Solid Edge part; units mm, degrees
sketch "Sketch1" plane through (0, 0, 0) normal (0, 0, 1) x (1, 0, 0)
  line L0 (-35, -27.5) -> (35, -27.5)
  line L1 (35, -27.5) -> (35, 27.5)
  line L2 (35, 27.5) -> (-35, 27.5)
  line L3 (-35, 27.5) -> (-35, -27.5)
extrude "Protrusion1" add sketch "Sketch1" along normal blind 1.6
sketch "Sketch2" plane through (0, 0, 0) normal (0, 0, 1) x (1, 0, 0)
  circle A0 centre (-31.5, -24) radius 1.5
  circle A1 centre (-31.5, 24) radius 1.5
  circle A2 centre (31.5, 24) radius 1.5
  circle A3 centre (31.5, -24) radius 1.5
extrude "Cutout1" cut sketch "Sketch2" along normal up to vertex (1.6 mm away)
sketch "Sketch3" plane through (0, 0, 1.6) normal (0, 0, 1) x (1, 0, 0)
  line L0 (-28, 17.5) -> (-46, 17.5)
  line L1 (-46, 17.5) -> (-46, 3.5)
  line L2 (-46, 3.5) -> (-28, 3.5)
  line L3 (-28, 3.5) -> (-28, 17.5)
extrude "ExtrudedProtrusion_2" add sketch "Sketch3" along normal blind 5
sketch "Sketch4" plane through (0, 0, 1.6) normal (0, 0, 1) x (1, 0, 0)
  line L0 (-35, -0.7) -> (-35, -9.7)
  line L1 (-35, -9.7) -> (-27.5, -9.7)
  line L2 (-27.5, -9.7) -> (-27.5, -0.7)
  line L3 (-27.5, -0.7) -> (-35, -0.7)
extrude "ExtrudedProtrusion_3" add sketch "Sketch4" along normal blind 3
sketch "Sketch5" plane through (0, 0, 1.6) normal (0, 0, 1) x (1, 0, 0)
  line L0 (25.5, -11.5) -> (-26.5, -11.5)
  line L1 (-26.5, -11.5) -> (-26.5, -24.5)
  line L2 (-26.5, -24.5) -> (25.5, -24.5)
  line L3 (25.5, -24.5) -> (25.5, -11.5)
extrude "ExtrudedProtrusion_4" add sketch "Sketch5" along normal blind 10
sketch "Sketch6" plane through (0, 0, 1.6) normal (0, 0, 1) x (1, 0, 0)
  line L0 (-23.5285, 7.5572) -> (-17.5285, 7.5572)
  line L1 (-17.5285, 7.5572) -> (-17.5285, 11.5572)
  line L2 (-17.5285, 11.5572) -> (-23.5285, 11.5572)
  line L3 (-23.5285, 11.5572) -> (-23.5285, 7.5572)
  line L4 (22.7373, -7.827) -> (22.7373, -3.827)
  line L5 (22.7373, -3.827) -> (16.7373, -3.827)
  line L6 (16.7373, -3.827) -> (16.7373, -7.827)
  line L7 (16.7373, -7.827) -> (22.7373, -7.827)
extrude "ExtrudedProtrusion_5" add sketch "Sketch6" along normal blind 2
sketch "Sketch7" plane through (0, 0, 1.6) normal (0, 0, 1) x (1, 0, 0)
  line L0 (13.5, 18.5) -> (-4.5, 18.5)
  line L1 (-4.5, 18.5) -> (-4.5, -7.5)
  line L2 (-4.5, -7.5) -> (13.5, -7.5)
  line L3 (13.5, -7.5) -> (13.5, 18.5)
extrude "ExtrudedProtrusion_6" add sketch "Sketch7" along normal blind 3
sketch "Sketch8" plane through (0, 0, 0) normal (0, 0, -1) x (-1, 0, 0)
  line L0 (26.5, -24.5) -> (-25.5, -24.5)
  line L1 (-25.5, -24.5) -> (-25.5, -11.5)
  line L2 (-25.5, -11.5) -> (26.5, -11.5)
  line L3 (26.5, -11.5) -> (26.5, -24.5)
extrude "ExtrudedProtrusion_7" add sketch "Sketch8" along normal blind 2
properties material "Polycarbonate"
Model file for the job. Use its own axes, mm. A direction names the side the tool comes from. Give positions to 0.01 mm unless a question says otherwise; leave off trailing zeros. Loops run counter-clockwise (first coordinate to the right, second up) from the corner with the lowest first, then second, coordinate; pieces in that order, holes last. Notation, with made-up numbers: M 49,-35 L 56,-35 A35 cw 56,3 Z; hole C 19.25,-13 d8. An arc over 180 degrees is marked long. Use one line per item in the form item = value.
Item 1: Slice it at A-A on x = 31.5. List the corners of the cut face in (y, z), and give its area (3 significant figures).
Filled in:
outline = M -27.5,0 L -25.5,0 L -25.5,1.6 L -27.5,1.6 Z; M -22.5,0 L 22.5,0 L 22.5,1.6 L -22.5,1.6 Z; M 25.5,0 L 27.5,0 L 27.5,1.6 L 25.5,1.6 Z
area = 78.4 mm^2
Item 2: Which spindle directions (+Z, -Z, +X, -X, +Y, -Y) get a long thin tool onto all of the face, cutting with end or side? Do faces 5 (the flat face through (20, -6, 3.6)), 6 (the flat face through (-28, 10, 4)), 7 (the flat face through (-31, -5, 4.6)), 8 (the flat face through (0, -11.5, -1)), 9 (the flat face through (-31, -0.7, 3)). Say none if no direction does.
Filled in:
face_5 = +Z, +X, +Y
face_6 = +Z, +Y
face_7 = +Z, +X, -X, -Y
face_8 = -Z, +X, -X, +Y
face_9 = +Z, -X
Item 3: Slice it at D-D on x = 3. List the corners of the cut face in (y, z).
Filled in:
outline = M -27.5,0 L -24.5,0 L -24.5,-2 L -11.5,-2 L -11.5,0 L 27.5,0 L 27.5,1.6 L 18.5,1.6 L 18.5,4.6 L -7.5,4.6 L -7.5,1.6 L -11.5,1.6 L -11.5,11.6 L -24.5,11.6 L -24.5,1.6 L -27.5,1.6 Z
Item 4: Slice it at B-B on y = 24. List the corners of the cut face in (x, z), and give its area (3 significant figures).
Filled in:
outline = M -35,0 L -33,0 L -33,1.6 L -35,1.6 Z; M -30,0 L 30,0 L 30,1.6 L -30,1.6 Z; M 33,0 L 35,0 L 35,1.6 L 33,1.6 Z
area = 102 mm^2
Item 5: Drill centre lines: L1, parallel to Y at x = -31.5, z = 0.65; L2, parallel to X at y = -7, z = 1.75; L3, parallel to X at y = 6, z = 3.5. Where is each one in solid material? Low to high.
Filled in:
L1 = -27.5 to -25.5, -22.5 to 22.5, 25.5 to 27.5
L2 = -35 to -27.5, -4.5 to 13.5, 16.74 to 22.74
L3 = -46 to -28, -4.5 to 13.5
Item 6: Flat gauge pins, fed straight in: pin 1 Ø6 at (x, y) = (-24.5, 1) entering from +Z; pin 2 Ø5.5 at (x, z) = (-40, 4.5) entering from -Y; pin 3 Ø6 at (x, y) = (10, 17.5) entering from -Z; pin 4 Ø2 at (y, z) = (-1.5, 6) entering from +X. Where does each tip first touch, or does it go through?
Filled in:
pin_1 = 1.6
pin_2 = 3.5
pin_3 = 0
pin_4 = through
Item 7: Two-plate mould, pull along X, no slides. Class faces 1 (the flat face through (-17.528, 10, 3)), 2 (the cylindrical face through (-32.61, 22.99, 0.79)), 3 (the flat face through (-26.5, -18, 7)), 4 (the flat face through (0, 27.5, 1)): released by +X, released by -X, zero draft, split by the parting line, or undercut.
Filled in:
face_1 = undercut
face_2 = undercut
face_3 = released by -X
face_4 = zero draft
Item 8: Slice it at C-C on z = 2.5. List the corners of the cut face in (x, y), and give its area (3 significant figures).
Filled in:
outline = M -46,3.5 L -28,3.5 L -28,17.5 L -46,17.5 Z; M -35,-9.7 L -27.5,-9.7 L -27.5,-0.7 L -35,-0.7 Z; M -26.5,-24.5 L 25.5,-24.5 L 25.5,-11.5 L -26.5,-11.5 Z; M -23.53,7.56 L -17.53,7.56 L -17.53,11.56 L -23.53,11.56 Z; M -4.5,-7.5 L 13.5,-7.5 L 13.5,18.5 L -4.5,18.5 Z; M 16.74,-7.83 L 22.74,-7.83 L 22.74,-3.83 L 16.74,-3.83 Z
area = 1,510 mm^2
